from build123d import *

# Parameters (mm, degrees)
SKETCH1_R           = 1.75
BOSS_EXTRUDE1_DEPTH = 3


with BuildPart() as part:
    # Sketch1 → Boss-Extrude1 (new body)
    with BuildSketch(Plane.XY):
        with BuildLine():
            Line((-69.999999999, 218.999999943), (-28.469288178, 218.999999943))
            Line((-28.469288178, 218.999999943), (-28.469288178, 190.499999944))
            ThreePointArc((-28.469288178, 190.499999944), (-28.176394959, 189.792893162), (-27.469288178, 189.499999944))
            Line((-27.469288178, 189.499999944), (27.510237275, 189.499999944))
            ThreePointArc((27.510237275, 189.499999944), (28.217344056, 189.792893162), (28.510237275, 190.499999944))
            Line((28.510237275, 190.499999944), (28.510237275, 219.000000001))
            Line((28.510237275, 219.000000001), (70, 219.000000001))
            ThreePointArc((70, 219.000000001), (62.928932188, 216.071067813), (60, 209.000000001))
            Line((60, 209.000000001), (60.000000001, 42.74629253))
            ThreePointArc((60.000000001, 42.74629253), (59.121320345, 40.624972187), (57.000000001, 39.74629253))
            Line((57.000000001, 39.74629253), (34.010726172, 39.74629253))
            add(Edge.make_bspline(
                [(19.726580347, 54.15000005), (28.313482135, 48.285383123), (34.010726172, 39.74629253)],
                knots=[0, 0, 0, 1, 1, 1], degree=2))
            Line((19.726580347, 54.15000005), (-19.726580417, 54.150000001))
            add(Edge.make_bspline(
                [(-34.010726207, 39.746292473), (-28.313482185, 48.285383067), (-19.726580417, 54.150000001)],
                knots=[0, 0, 0, 1, 1, 1], degree=2))
            Line((-34.010726207, 39.746292473), (-56.999999999, 39.746292473))
            ThreePointArc((-56.999999999, 39.746292473), (-59.121320343, 40.624972129), (-59.999999999, 42.746292473))
            Line((-59.999999999, 42.746292473), (-59.999999999, 208.999999944))
            ThreePointArc((-59.999999999, 208.999999944), (-62.928932187, 216.071067755), (-69.999999999, 218.999999943))
        make_face()
        with Locations((-50, 189)):
            Circle(SKETCH1_R, mode=Mode.SUBTRACT)
        with Locations((50, 189.000000001)):
            Circle(SKETCH1_R, mode=Mode.SUBTRACT)
        with Locations((-49.999999999, 64.74629253)):
            Circle(SKETCH1_R, mode=Mode.SUBTRACT)
        with Locations((50.000000001, 64.74629253)):
            Circle(SKETCH1_R, mode=Mode.SUBTRACT)
    extrude(amount=BOSS_EXTRUDE1_DEPTH)


solid = part.part
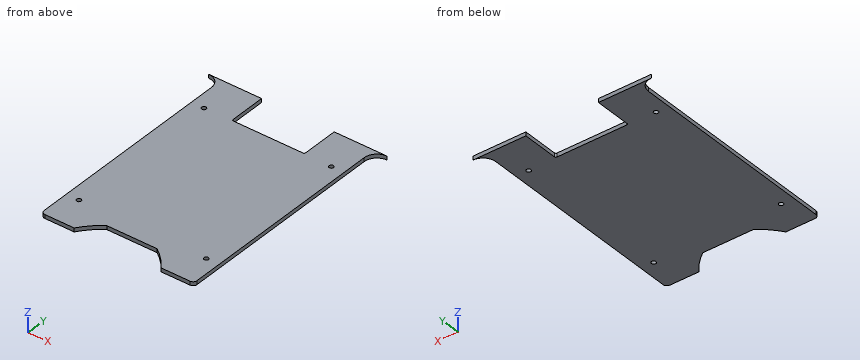
Can you work these out from the model? Positions are in its coordinate system, mm. Give positions to 0.01 mm unless a question says otherwise; leave off trailing zeros. Loops run counter-clockwise (first coordinate to the right, second up) from the corner with the lowest first, then second, coordinate; pieces in that order, holes last. Notation, with made-up numbers: (8.5, -35) - (38.5, -35) arc R15 cw to (38.5, -6) - close; hole circle Ø6 at (65, 49). An arc over 180 degrees is marked (long way). Answer as a JSON object with one key per item and string values.
Q1. If I drill on L1, parallel to Y at x = 50, z = 1.15; L2, parallel to X at y = 62, z = 0.95; L3, parallel to Y at x = 9, z = 2.65, over which ranges is the centre line in solid material (lowest first)?
Geometry says:
{"L1": "39.75 to 63, 66.5 to 187.25, 190.75 to 219", "L2": "-60 to 60", "L3": "54.15 to 189.5"}
Q2. Will these pins go through, and if not, where does the flat tip stop? P1, Ø0.9, axis at y = 198.5, z = 1.5, coming from the -X side; P2, Ø0.9, axis at y = 201, z = 1, coming from the +X side; P3, Ø0.9, axis at x = -6.5, z = 1, coming from the +Y side; P4, Ø2, axis at x = -50, y = 189, coming from the -Z side.
Geometry says:
{"P1": "x = -60", "P2": "x = 60", "P3": "y = 189.5", "P4": "through"}
Q3. Imagine slicing it at A-A on y = 193. Write out the boundary of the cut face in (x, z), plus the area to 3 significant figures.
Geometry says:
{"outline": "(-60, 0) - (-28.47, 0) - (-28.47, 3) - (-60, 3) - close; (28.51, 0) - (60, 0) - (60, 3) - (28.51, 3) - close", "area": "189 mm²"}
Q4. Imagine slicing it at D-D on z = 2.15. Give the number of separate pieces and of enclosed holes in the cut face, plus the area to 3 significant figures.
Geometry says:
{"separate pieces": "1", "enclosed holes": "4", "area": "19,000 mm²"}
Q5. Imagine slicing it at C-C on y = 159.5. Write out the boundary of the cut face in (x, z).
Geometry says:
{"outline": "(-60, 0) - (60, 0) - (60, 3) - (-60, 3) - close"}
Q6. Imagine slicing it at B-B on x = -8. Write out the boundary of the cut face in (y, z), plus the area to 3 significant figures.
Geometry says:
{"outline": "(54.15, 0) - (189.5, 0) - (189.5, 3) - (54.15, 3) - close", "area": "406 mm²"}
